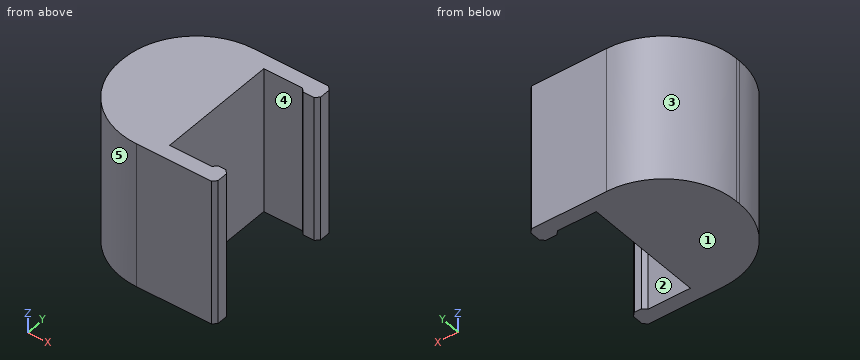
```python
from build123d import *

# Parameters (mm, degrees)
F0_W     = 5.8
F0_H     = 2
F1_DEPTH = 20
F2_R     = 10
F3_SIZE  = 0.49999


# Not quite as in the source:
# - a fillet or chamfer is up to 0.001 mm smaller than in the source, because OpenCascade refuses the exact size


with BuildPart() as f1:
    # F0 (on Top) → F1 (new body)
    with BuildSketch(Plane.XY):
        with Locations((-51.9097009659, 46.350823313)):
            Rectangle(F0_W, F0_H)
        Polygon((-54.8097009659, 45.350823313), (-54.8097009659, 47.350823313), (-67.8097009659, 47.350823313), (-67.8097009659, 26.850823313), (-54.8097009659, 26.850823313), (-54.8097009659, 28.850823313), align=None)
        Polygon((-47.0097009659, 47.350823313), (-49.0097009659, 47.350823313), (-49.0097009659, 45.350823313), (-49.0097009659, 44.850823313), (-47.0097009659, 44.850823313), align=None)
        with Locations((-51.9097009659, 27.850823313)):
            Rectangle(F0_W, F0_H)
        Polygon((-49.0097009659, 29.350823313), (-49.0097009659, 28.850823313), (-49.0097009659, 26.850823313), (-47.0097009659, 26.850823313), (-47.0097009659, 29.350823313), align=None)
    extrude(amount=F1_DEPTH)

    # F2
    f2_edges = [f1.edges().sort_by_distance(p)[0] for p in [
        (-67.809701, 47.350823, 10),
        (-67.809701, 26.850823, 10),
    ]]
    fillet(f2_edges, radius=F2_R)

    # F3 (size 0.5 in the source; OpenCascade refuses exactly that, so slightly less here)
    f3_edges = [f1.edges().sort_by_distance(p)[0] for p in [
        (-47.009701, 47.350823, 10),
        (-47.009701, 44.850823, 10),
        (-47.009701, 29.350823, 10),
        (-47.009701, 26.850823, 10),
        (-49.009701, 29.350823, 10),
        (-49.009701, 45.350823, 10),
    ]]
    chamfer(f3_edges, length=F3_SIZE)


solid = f1.part
```
Check sheet for the modelled part. Datum: model origin and axes. Units: mm. Face numbers are marked on the shaded views. A direction names the side the tool comes from. Give positions to 0.01 mm unless a question says otherwise; leave off trailing zeros. Loops run counter-clockwise (first coordinate to the right, second up) from the corner with the lowest first, then second, coordinate; pieces in that order, holes last. Notation, with made-up numbers: (26.5, -6) - (82.5, -6) arc R13 ccw to (82.5, 6) - close; hole circle Ø3 at (-12, -4). An arc over 180 degrees is marked (long way). One line per question, with ' | ' between items. Start each with the question number.
1. Draft check along Y on the marked faces 3, 4 and 5. Enter one of: released by +Y, released by -Y, zero draft, split by the parting line, or undercut.
2. Set-up check for the marked faces 1 and 2: record each of +Z, -Z, +X, -X, +Y, -Y from which the full face is reachable in a straight line by a thin tool's end or side.
3. Cross-section at D-D, the plane x = -66.5. Enter the section's corners in (y, z), plus the area to 3 significant figures.
4. Cross-section at A-A, the plane x = -50.75. Enter the section's corners in (y, z), plus the area to 3 significant figures.
5. Cross-section at C-C, the plane y = 42.5. Enter the section's corners in (x, z).
6. Material ranges on line 1 along Y through (x, z) = (-54, 18.5); line 2 along Y through (x, z) = (-48, 5.25); line 3 along X through (y, z) = (36.75, 13.5), recorded low to high. Write a range as [from, to].
7. Gauge pin test, flat ends, axial feed: pin 1 Ø4 at (x, y) = (-52, 40) entering from +Z (1 decimal); pin 2 Ø8 at (y, z) = (30.5, 14) entering from -X; pin 3 Ø5 at (x, z) = (-65.5, 10.5) entering from -Y. Record the tip position at first contact, or that the pin passes through.
Check result:
1) face 3: released by +Y | face 4: undercut | face 5: released by -Y
2) face 1: -Z, +X, -X, +Y, -Y | face 2: +Z, -Z
3) outline: (31.9, 0) - (42.3, 0) - (42.3, 20) - (31.9, 20) - close | area: 208 mm2
4) outline: (26.85, 0) - (28.85, 0) - (28.85, 20) - (26.85, 20) - close; (45.35, 0) - (47.35, 0) - (47.35, 20) - (45.35, 20) - close | area: 80.0 mm2
5) outline: (-66.38, 0) - (-54.81, 0) - (-54.81, 20) - (-66.38, 20) - close
6) line 1: y = [26.85, 28.85], [45.35, 47.35] | line 2: y = [26.85, 29.35], [44.85, 47.35] | line 3: x = [-67.81, -54.81]
7) pin 1: passes through | pin 2: stops at x = -67.53 | pin 3: stops at y = 28.3
